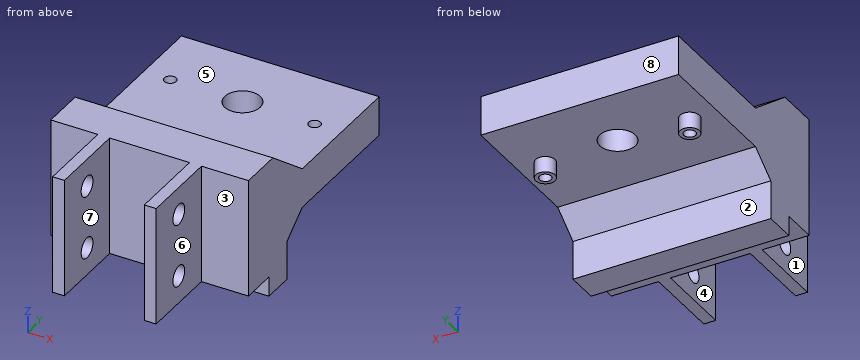
```python
from build123d import *

# Parameters (mm, degrees)
EXTRUDE_1_DEPTH     = 30
SKETCH_2_W          = 50
SKETCH_2_H          = 10
EXTRUDE_2_DEPTH     = 50
HOLE_WIZARD_2_D     = 5.2
HOLE_WIZARD_3_D     = 9
SKETCH_17_R         = 2.45
EXTRUDE_6_DEPTH     = 4
HOLE_WIZARD_5_D     = 3
EXTRUDE_7_DEPTH     = 50
SKETCH_21_W         = 10
SKETCH_21_H         = 3
CUT_EXTRUDE_1_DEPTH = 81.413870849
SKETCH_23_W         = 9.807692308
SKETCH_23_H         = 8
EXTRUDE_8_DEPTH     = 50


with BuildPart() as part:
    # 草图1 → 凸台-拉伸1 (new body)
    with BuildSketch(Plane.XY):
        Polygon((13.1, -5.375), (13.1, -25.375), (10.1, -25.375), (10.1, -5.375), (-10.1, -5.375), (-10.1, -25.375), (-13.1, -25.375), (-13.1, -5.375), (-25, -5.375), (-25, 5.375), (25, 5.375), (25, -5.375), align=None)
    extrude(amount=EXTRUDE_1_DEPTH)

    # 草图2 → 凸台-拉伸2 (add)
    with BuildSketch(Plane(origin=(0, 5.375, 0), x_dir=(1, 0, 0), z_dir=(0, 1, 0))):
        with Locations((0, -15)):
            Rectangle(SKETCH_2_W, SKETCH_2_H)
    extrude(amount=EXTRUDE_2_DEPTH)

    # 孔2 (through all)
    with Locations(Plane.ZY.offset(13.1)):
        with Locations((7, -15.375), (23, -15.375)):
            Hole(HOLE_WIZARD_2_D / 2)

    # 孔3 (through all)
    with Locations(Plane(origin=(0, 0, 10), x_dir=(-1, 0, 0), z_dir=(0, 0, -1))):
        with Locations((0, 35.625)):
            Hole(HOLE_WIZARD_3_D / 2)

    # 草图17 → 凸台-拉伸6 (add)
    with BuildSketch(Plane(origin=(0, 0, 10), x_dir=(-1, 0, 0), z_dir=(0, 0, -1))):
        with Locations(Location((18.25, 35.625, 0), (0, 0, 180))):
            Circle(SKETCH_17_R)
        with Locations(Location((-18.25, 35.625, 0), (0, 0, 180))):
            Circle(SKETCH_17_R)
    extrude(amount=EXTRUDE_6_DEPTH)

    # 孔5 (through all)
    with Locations(Plane(origin=(0, 0, 6), x_dir=(-1, 0, 0), z_dir=(0, 0, -1))):
        with Locations((18.25, 35.625), (-18.25, 35.625)):
            Hole(HOLE_WIZARD_5_D / 2)

    # 草图20 → 凸台-拉伸7 (add)
    with BuildSketch(Plane.ZY.offset(25)):
        Polygon((20, 18.375), (30, 5.375), (20, 5.375), align=None)
        Polygon((10, 18.375), (0, 5.375), (10, 5.375), align=None)
    extrude(amount=-EXTRUDE_7_DEPTH)

    # 草图21 → 切除-拉伸1 (cut, through all)
    with BuildSketch(Plane.ZY.offset(25)):
        with Locations((15, 53.875)):
            Rectangle(SKETCH_21_W, SKETCH_21_H)
    extrude(amount=-CUT_EXTRUDE_1_DEPTH, mode=Mode.SUBTRACT)

    # 草图23 → 凸台-拉伸8 (add)
    with BuildSketch(Plane(origin=(25, 0, 0), x_dir=(0, 0, -1), z_dir=(1, 0, 0))):
        with Locations((0.096153846, 7.625)):
            Rectangle(SKETCH_23_W, SKETCH_23_H)
    extrude(amount=-EXTRUDE_8_DEPTH)


solid = part.part
```
The listing builds one solid part. Answer for the finished solid, in the listing's coordinates (mm). Face numbers are marked on the shaded views. A direction names the side the tool comes from. Coordinates: 2 decimals unless noted, no trailing zeros. Write each loop counter-clockwise with the first axis right and the second up, starting at its lowest first coordinate (ties: lowest second). Pieces come first, ordered by that corner, then holes. Notation, with made-up numbers: (10, 80) - (42, 80) arc R18 ccw to (42, 84) - close; hole circle Ø8 at (85, 77). An arc over 180 degrees is marked (long way). Return JSON: item names as keys, results as strings. Group by question number.
Q1. The part is cut by section B-B on z = 7. Write down the section's boundary in (x, y) (3 decimals).
Q2. The part is cut by section A-A on x = -18.25. Write down the section's boundary in (y, z) (3 decimals), and give its area (3 significant figures).
Q3. The part is cut by section D-D on y = -14. Write down the section's boundary in (x, z), and give its area (3 significant figures).
Q4. Find the intervals of material crossed by line 1 along Y through (x, z) = (18.25, 12.75) (3 decimals); line 2 along Z through (x, y) = (-18.5, 1); line 3 along Z through (x, y) = (-20.5, 46), in increasing order. Write a range as [from, to].
Q5. The part is cut by section C-C on y = 32. Write down the section's boundary in (x, z), and give its area (3 significant figures).
Q6. Which of the six approach directions +Z, -Z, +X, -X, +Y, -Y give full straight-line access (tool end or side, diameter ignored) to the marked faces 1, 2, 3, 4 and 5?
Q7. For a pull along X with two mould halves and no side action, classify the marked faces 6, 7 and 8 as +X half, -X half, draft (parallel to the pull), parting line (faces both ways), or undercut.
Q8. Flat-ended cylindrical pins translate along their axes: pin 1 Ø10 at (y, z) = (27, -1) entering from -X; pin 2 Ø6 at (y, z) = (-15.375, 23) entering from +X; pin 3 Ø1.5 at (y, z) = (33.5, 7.5) entering from -X; pin 4 Ø4 at (x, y) = (7.5, 19.5) entering from -Z. Find the tip coordinate at first contact, or state that the pin passes through.
Evaluation:
{
 "1": {"outline": "(-25, -5.375) - (-13.1, -5.375) - (-13.1, -12.775) - (-10.1, -12.775) - (-10.1, -5.375) - (10.1, -5.375) - (10.1, -12.775) - (13.1, -12.775) - (13.1, -5.375) - (25, -5.375) - (25, 14.475) - (-25, 14.475) - close; circle Ø4.9 at (-18.25, 35.625); (-13.1, -25.375) - (-10.1, -25.375) - (-10.1, -17.975) - (-13.1, -17.975) - close; (10.1, -25.375) - (13.1, -25.375) - (13.1, -17.975) - (10.1, -17.975) - close; circle Ø4.9 at (18.25, 35.625); hole circle Ø3 at (-18.25, 35.625); hole circle Ø3 at (18.25, 35.625)"},
 "2": {"outline": "(-5.375, 0) - (3.625, 0) - (3.625, -5) - (11.625, -5) - (11.625, 4.808) - (18.375, 10) - (33.175, 10) - (33.175, 6) - (34.125, 6) - (34.125, 20) - (18.375, 20) - (5.375, 30) - (-5.375, 30) - close; (37.125, 6) - (38.075, 6) - (38.075, 10) - (52.375, 10) - (52.375, 20) - (37.125, 20) - close", "area": "955 mm2"},
 "3": {"outline": "(-13.1, 0) - (-10.1, 0) - (-10.1, 4.79) - (-13.1, 4.79) - close; (-13.1, 9.21) - (-10.1, 9.21) - (-10.1, 20.79) - (-13.1, 20.79) - close; (-13.1, 25.21) - (-10.1, 25.21) - (-10.1, 30) - (-13.1, 30) - close; (10.1, 0) - (13.1, 0) - (13.1, 4.79) - (10.1, 4.79) - close; (10.1, 9.21) - (13.1, 9.21) - (13.1, 20.79) - (10.1, 20.79) - close; (10.1, 25.21) - (13.1, 25.21) - (13.1, 30) - (10.1, 30) - close", "area": "127 mm2"},
 "4": {"line 1": "y = [-5.375, 34.125], [37.125, 52.375]", "line 2": "z = [0, 30]", "line 3": "z = [10, 20]"},
 "5": {"outline": "(-25, 10) - (-2.67, 10) - (-2.67, 20) - (-25, 20) - close; (2.67, 10) - (25, 10) - (25, 20) - (2.67, 20) - close", "area": "447 mm2"},
 "6": {"face 1": "+Z, -Z, -X, -Y", "face 2": "-Z, +X, -X, +Y", "face 3": "+Z, -Z, +X, -Y", "face 4": "+Z, -Z, -Y", "face 5": "+Z, +X, -X, +Y"},
 "7": {"face 6": "+X half", "face 7": "undercut", "face 8": "draft"},
 "8": {"pin 1": "passes through", "pin 2": "stops at x = 13.1", "pin 3": "stops at x = -20.28", "pin 4": "stops at z = 9.33"}
}
